Check sheet for the modelled part. Datum: model origin and axes. Units: mm. Face numbers are marked on the shaded views. A direction names the side the tool comes from. Coordinates: 2 decimals unless noted, no trailing zeros. Order: outer loops, then holes, each group sorted by start corner. A loop starts at its lowest first (then second) coordinate and runs counter-clockwise, first axis right, second up.
1. Set-up check for the marked faces 1, 2 and 3: record each of +Z, -Z, +X, -X, +Y, -Y from which the full face is reachable in a straight line by a thin tool's end or side.
2. Thickness scan on line 1 (Y direction, x = 11.5, z = 105); line 2 (X direction, y = -24, z = 147); line 3 (Z direction, x = 39, y = -22.5). Record the ranges inside material, lowest first.
3. Cross-section at A-A (y = -20). Enter the section's corners in (x, z), then the cut area to 3 significant figures.
4. Cross-section at C-C (z = 61). Enter the section's corners in (x, y), then the cut area to 3 significant figures.
5. Cross-section at B-B (x = 21). Count the separate pieces of the cut face and the enclosed holes in it, then the cut area to 3 significant figures.
6. Gauge pin test, flat ends, axial feed: pin 1 Ø1.8 at (x, z) = (40.5, 48.5) entering from +Y; pin 2 Ø5 at (x, y) = (25.5, 14) entering from -Z; pin 3 Ø18 at (x, z) = (14.5, 54.5) entering from -Y; pin 4 Ø12.5 at (x, y) = (27.5, 43.5) entering from +Z. Record the tip position at first contact, or that the pin passes through.
7. Cross-section at D-D (y = 39). Enter the section's corners in (x, z).
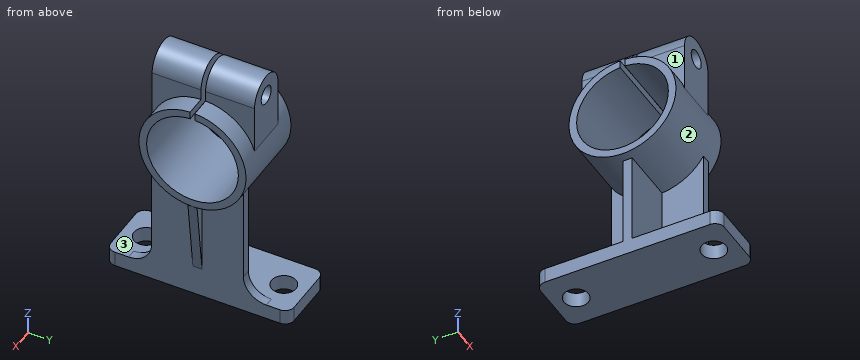
```python
from build123d import *

# Parameters (mm, degrees)
PAD_DEPTH       = 42
SKETCH001_W     = 57
SKETCH001_H     = 36
POCKET_DEPTH    = 95
FILLET_R        = 6
FILLET001_R     = 6
FILLET002_R     = 6
FILLET003_R     = 6
SKETCH002_R     = 8
POCKET001_DEPTH = 10.001
POCKET002_DEPTH = 42.001
SKETCH004_R     = 35
PAD001_DEPTH    = 54
PAD002_DEPTH    = 33.5
POCKET003_DEPTH = 54.001
SKETCH008_R     = 6
POCKET004_DEPTH = 93.501
PAD003_DEPTH    = 3


with BuildPart() as part:
    # Sketch → Pad (new body)
    with BuildSketch(Plane.YZ):
        with BuildLine():
            Line((-60, 0), (60, 0))
            Line((60, 0), (60, 10))
            Line((60, 10), (45, 10))
            ThreePointArc((30, 25), (34.393398, 14.393398), (45, 10))
            Line((30, 25), (30, 105))
            Line((30, 105), (-30, 105))
            Line((-30, 105), (-30, 25))
            ThreePointArc((-45, 10), (-34.393398, 14.393398), (-30, 25))
            Line((-45, 10), (-60, 10))
            Line((-60, 10), (-60, 0))
        make_face()
    extrude(amount=PAD_DEPTH)

    # Sketch001 (on Face8 of Pad) → Pocket (cut)
    with BuildSketch(Plane(origin=(0, 0, 105), x_dir=(0, -1, 0), z_dir=(0, 0, 1))):
        with Locations((-31.5, 18)):
            Rectangle(SKETCH001_W, SKETCH001_H)
        with Locations((31.5, 18)):
            Rectangle(SKETCH001_W, SKETCH001_H)
    extrude(amount=-POCKET_DEPTH, mode=Mode.SUBTRACT)

    # Fillet
    fillet_edges = [part.edges().sort_by_distance(p)[0] for p in [
        (42, -60, 5),
    ]]
    fillet(fillet_edges, radius=FILLET_R)

    # Fillet001
    fillet001_edges = [part.edges().sort_by_distance(p)[0] for p in [
        (0, -60, 5),
    ]]
    fillet(fillet001_edges, radius=FILLET001_R)

    # Fillet002
    fillet002_edges = [part.edges().sort_by_distance(p)[0] for p in [
        (42, 60, 5),
    ]]
    fillet(fillet002_edges, radius=FILLET002_R)

    # Fillet003
    fillet003_edges = [part.edges().sort_by_distance(p)[0] for p in [
        (0, 60, 5),
    ]]
    fillet(fillet003_edges, radius=FILLET003_R)

    # Sketch002 (on Face14 of Fillet003) → Pocket001 (cut, through all)
    with BuildSketch(Plane(origin=(0, 0, 10), x_dir=(0, -1, 0), z_dir=(0, 0, 1))):
        with Locations((-45, 21)):
            Circle(SKETCH002_R)
        with Locations((45, 21)):
            Circle(SKETCH002_R)
    extrude(amount=-POCKET001_DEPTH, mode=Mode.SUBTRACT)

    # Sketch003 → Pocket002 (cut, through all)
    with BuildSketch(Plane.YZ):
        with BuildLine():
            ThreePointArc((-35, 105), (0, 70), (35, 105))
            Line((-35, 105), (35, 105))
        make_face()
    extrude(amount=POCKET002_DEPTH, mode=Mode.SUBTRACT)

    # Sketch004 → Pad001 (join)
    with BuildSketch(Plane(origin=(48, 0, 105), x_dir=(0, 0, -1), z_dir=(1, 0, 0))):
        Circle(SKETCH004_R)
    extrude(amount=-PAD001_DEPTH)

    # Sketch006 → Pad002 (join, symmetric)
    with BuildSketch(Plane.XZ):
        with BuildLine():
            Line((7, 146.999962), (7, 104.999962))
            Line((7, 104.999962), (35, 105))
            Line((35, 105), (35, 146.999962))
            ThreePointArc((35, 146.999962), (21, 160.999962), (7, 146.999962))
        make_face()
    extrude(amount=PAD002_DEPTH, both=True)

    # Sketch007 (on Face28 of Pad002) → Pocket003 (cut, through all)
    with BuildSketch(Plane.YZ.offset(48)):
        with BuildLine():
            ThreePointArc((-1.5, 134.962477), (0, 75), (1.5, 134.962477))
            Line((1.5, 163), (1.5, 134.962477))
            Line((-1.5, 163), (1.5, 163))
            Line((-1.5, 134.962477), (-1.5, 163))
        make_face()
    extrude(amount=-POCKET003_DEPTH, mode=Mode.SUBTRACT)

    # Sketch008 (on Face30 of Pocket003) → Pocket004 (cut, through all)
    with BuildSketch(Plane(origin=(0, -33.5, 0), x_dir=(0, 0, -1), z_dir=(0, -1, 0))):
        with Locations((-147, 21)):
            Circle(SKETCH008_R)
    extrude(amount=-POCKET004_DEPTH, mode=Mode.SUBTRACT)

    # Sketch009 → Pad003 (join, symmetric)
    with BuildSketch(Plane.XZ):
        Polygon((42, 70), (42, 20), (48, 70), align=None)
    extrude(amount=PAD003_DEPTH, both=True)


solid = part.part
```
Data:
1. face 1: +Z, -X, -Y
1. face 2: none
1. face 3: -X, -Y
2. line 1: y = -35 to -30, 30 to 35
2. line 2: x = 7 to 15, 27 to 35
2. line 3: z = 0 to 85.16, 124.84 to 131.81
3. outline: (-6, 76.28) - (36, 76.28) - (36, 10) - (0, 10) - (0, 0) - (42, 0) - (42, 76.28) - (48, 76.28) - (48, 82.64) - (-6, 82.64) - close; (-6, 127.36) - (48, 127.36) - (48, 133.72) - (35, 133.72) - (35, 147) arc R14 ccw to (7, 147) - (7, 133.72) - (-6, 133.72) - close; hole circle Ø12 at (21, 147)
3. area: 2,070 mm2
4. outline: (0, -3) - (36, -3) - (36, -30) - (42, -30) - (42, -3) - (46.92, -3) - (46.92, 3) - (42, 3) - (42, 30) - (36, 30) - (36, 3) - (0, 3) - close
4. area: 606 mm2
5. separate pieces: 5
5. enclosed holes: 0
5. area: 3,260 mm2
6. pin 1: stops at y = 30
6. pin 2: stops at z = 0
6. pin 3: stops at y = -3
6. pin 4: stops at z = 10
7. outline: (0, 0) - (15.71, 0) - (15.71, 10) - (0, 10) - close; (26.29, 0) - (42, 0) - (42, 11.25) - (36, 11.25) - (36, 10) - (26.29, 10) - close
